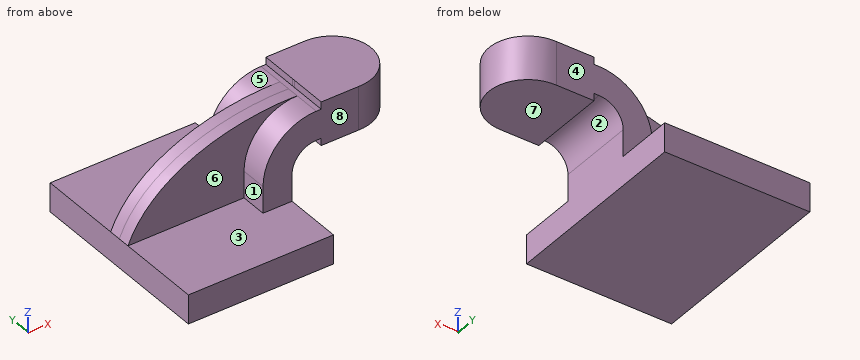
```python
from build123d import *

# Parameters (mm, degrees)
F1_DEPTH = 63.5
F2_DEPTH = 25.4
F3_DEPTH = 25.4
F4_DEPTH = 7.9375
F0_W     = 25.4115133166
F0_H     = 28.575


with BuildPart() as f1:
    # F0 (on Front) → F1 (new body, symmetric)
    with BuildSketch(Plane.XZ):
        Polygon((28.575, 9.525), (-47.625, 9.525), (-47.625, -9.525), (47.625, -9.525), (47.625, 9.525), align=None)
    extrude(amount=F1_DEPTH, both=True)

    # F0 (on Front) → F2 (join, symmetric)
    with BuildSketch(Plane.XZ):
        with BuildLine():
            Line((28.575, 27.0002), (28.575, 9.525))
            Line((28.575, 9.525), (47.625, 9.525))
            Line((47.625, 9.525), (47.625, 27.0002))
            ThreePointArc((47.625, 27.0002), (52.2746798487, 38.2255201513), (63.5, 42.8752))
            Line((63.5, 42.8752), (66.754385829, 42.8752))
            Line((66.754385829, 42.8752), (66.754385829, 61.9252))
            Line((66.754385829, 61.9252), (63.5, 61.9252))
            ThreePointArc((63.5, 61.9252), (38.8042956671, 51.6959043329), (28.575, 27.0002))
        make_face()
    extrude(amount=F2_DEPTH, both=True)

    # F0 (on Front) → F3 (join, symmetric)
    with BuildSketch(Plane.XZ):
        Polygon((66.754385829, 66.675), (66.754385829, 61.9252), (66.754385829, 42.8752), (66.754385829, 38.1), (92.1428725123, 38.1), (92.1428725123, 66.675), align=None)
    extrude(amount=F3_DEPTH, both=True)

    # F0 (on Front) → F4 (join, symmetric)
    with BuildSketch(Plane.XZ):
        with BuildLine():
            add(Edge.make_bspline(
                [(-47.625, 9.525), (-30.3663147909, 50.6522115959), (25.7086480849, 63.3923630702), (63.5, 61.9252)],
                knots=[0, 0, 0, 0, 122.8598656398, 122.8598656398, 122.8598656398, 122.8598656398], degree=3))
            Line((-47.625, 9.525), (28.575, 9.525))
            Line((28.575, 9.525), (28.575, 27.0002))
            ThreePointArc((28.575, 27.0002), (38.8042956671, 51.6959043329), (63.5, 61.9252))
        make_face()
    extrude(amount=F4_DEPTH, both=True)

    # F0 (on Front) → F5 (revolve)
    with BuildSketch(Plane.XZ):
        with Locations((104.8486291707, 52.3875)):
            Rectangle(F0_W, F0_H)
    revolve(axis=Axis((92.1428725123, 0, 52.3875), (0, 0, 1)))


solid = f1.part
```
Design review of the part built by this model. Coordinates are the model's own, in mm. Face numbers are marked on the shaded views. A direction names the side the tool comes from. Give positions to 0.01 mm unless a question says otherwise; leave off trailing zeros. Order: outer loops, then holes, each group sorted by start corner. A loop starts at its lowest first (then second) coordinate and runs counter-clockwise, first axis right, second up. Notation, with made-up numbers: (-2.5, 39) -> (1.5, 39) arc R15 ccw to (1.5, 60) -> close; hole circle Ø10 at (-8.75, 70). An arc over 180 degrees is marked (long way). Write item = value, one per line. Start each with the question number.
(1) For the marked faces 4, 5, 6, 7 and 8, list the 3-axis set-ups (+Z, -Z, +X, -X, +Y, -Y) from which the entire face can be reached by the end or side of a thin tool; tool diameter is ignored.
(2) For pin 1 (16 mm diameter, centred on x = -9, z = 37.5, fed in from +Y); pin 2 (1 mm diameter, centred on x = -29.5, y = -48.5, fed in from +Z) (3 decimals); pin 3 (2.5 mm diameter, centred on x = 65, y = -9, fed in from -Z), all flat-tipped, find the tip position at first contact; note any pin that passes through.
(3) Mouldability with a two-part tool opening along X and no side actions: class the marked faces 1, 2 and 3 as +X half, -X half, draft (parallel to the pull), parting line (faces both ways), or undercut.
(4) We need section A-A on z = 3.5. Write out the cut boundary in (x, y) (3 decimals).
(5) We need section C-C on y = 50. Write out the cut boundary in (x, z) (3 decimals), plus the area to 3 significant figures.
(6) We need section B-B on y = 10.5. Write out the cut boundary in (x, z) (3 decimals).
(7) To check wall thickness, follow line 1 along Z through (x, y) = (6.5, -34) (3 decimals); line 2 along Y through (x, z) = (23, 57); line 3 along Y through (x, z) = (49, 50.5). State the ranges of each line that lie inside material, in increasing order.
Numbers:
q1.face_4 = +Z, +X, -X, +Y
q1.face_5 = +Z, -X, +Y
q1.face_6 = +Z, -X, -Y
q1.face_7 = -Z, +X, +Y, -Y
q1.face_8 = +Z, +X, -X, -Y
q2.pin_1 = 7.94
q2.pin_2 = 9.525
q2.pin_3 = 42.88
q3.face_1 = -X half
q3.face_2 = undercut
q3.face_3 = draft
q4.outline = (-47.625, -63.5) -> (47.625, -63.5) -> (47.625, 63.5) -> (-47.625, 63.5) -> close
q5.outline = (-47.625, -9.525) -> (47.625, -9.525) -> (47.625, 9.525) -> (-47.625, 9.525) -> close
q5.area = 1,810 mm^2
q6.outline = (-47.625, -9.525) -> (47.625, -9.525) -> (47.625, 27) arc R15.875 cw to (63.5, 42.875) -> (66.754, 42.875) -> (66.754, 38.1) -> (115.284, 38.1) -> (115.284, 66.675) -> (66.754, 66.675) -> (66.754, 61.925) -> (63.5, 61.925) arc R34.925 ccw to (28.575, 27) -> (28.575, 9.525) -> (-47.625, 9.525) -> close
q7.line_1 = -9.525 to 9.525
q7.line_2 = -7.94 to 7.94
q7.line_3 = -25.4 to 25.4
